For this review, take the finished solid that the model builds, in its own axes (mm). Face numbers are marked on the shaded views. Round coordinates to 2 decimals unless told otherwise and drop trailing zeros. Write each loop counter-clockwise with the first axis right and the second up, starting at its lowest first coordinate (ties: lowest second). Pieces come first, ordered by that corner, then holes. Notation, with made-up numbers: M 48,76 L 66,76 A8 cw 66,89 Z; hole C -5.75,56.5 d4. An arc over 180 degrees is marked long. Use one line per item in the form item = value. Start each with the question number.
Item 1: Add section C-C (z = 11). State the section outline as (x, y) points, and give its area (3 significant figures).
Item 2: For line 1 (Z direction, x = 0, y = 3.1); line 2 (Z direction, x = 10.75, y = -4); line 3 (X direction, y = 0.5, z = 0.5), list the stretches that pass through material, from the lowest coordinate up. Write a range as [from, to].
Item 3: Add section B-B (y = -15.5). State the section outline as (x, z) points, and give its area (3 significant figures).
Item 4: Add section A-A (x = 0). State the section outline as (y, z) points (3 decimals).
Item 5: Draft analysis for pull direction Z (two halves, no side actions). For the marked faces 1 and 2, state which applies: released by +Z, released by -Z, zero draft, split by the parting line, or undercut.
Item 6: For P1, Ø3, axis at x = -2, y = -6, coming from the +Z side; P2, Ø1.5, axis at x = 8.5, y = 6.5, coming from the +Z side; P3, Ø8, axis at x = -0.5, z = 17, coming from the -Y side, all flat-tipped, find the tip position at first contact; note any pin that passes through.
from build123d import *

# Parameters (mm, degrees)
F2_DEPTH = 3.175
F0_R     = 6.35
F3_DEPTH = 3.175
F4_DEPTH = 19.05
F0_W     = 6.35
F0_H     = 25.4
F6_DEPTH = 3.048


with BuildPart() as f1:
    # F0 (on Front) → F1 (revolve)
    with BuildSketch(Plane.XZ):
        Polygon((12.7, 93.701775), (0, 93.701775), (0, -7.898225), (6.35, -7.898225), (12.7, -7.898225), align=None)
    revolve(axis=Axis((0, 0, 42.901775), (0, 0, -1)))

    # F0 (on Front) → F2 (join, symmetric)
    with BuildSketch(Plane.XZ):
        with BuildLine():
            Line((-9.525, 144.402459), (-12.7, 93.701775))
            Line((-12.7, 93.701775), (0, 93.701775))
            Line((0, 93.701775), (12.7, 93.701775))
            Line((12.7, 93.701775), (9.525, 144.402459))
            ThreePointArc((9.525, 144.402459), (0, 134.877459), (-9.525, 144.402459))
        make_face()
    extrude(amount=F2_DEPTH, both=True)

    # F0 (on Front) → F3 (join, symmetric)
    with BuildSketch(Plane.XZ):
        with BuildLine():
            ThreePointArc((9.525, 144.402459), (0, 153.927459), (-9.525, 144.402459))
            ThreePointArc((-9.525, 144.402459), (0, 134.877459), (9.525, 144.402459))
        make_face()
        with Locations((0, 144.402459)):
            Circle(F0_R, mode=Mode.SUBTRACT)
    extrude(amount=F3_DEPTH, both=True)

    # F0 (on Front) → F4 (join)
    with BuildSketch(Plane.XZ):
        with Locations((0, 144.402459)):
            Circle(F0_R)
    extrude(amount=F4_DEPTH)

    # F0 (on Front) → F5 (revolve)
    with BuildSketch(Plane.XZ):
        with Locations((3.175, -20.598225)):
            Rectangle(F0_W, F0_H)
    revolve(axis=Axis((0, 0, -20.598225), (0, 0, -1)))

    # F0 (on Front) → F6 (join)
    with BuildSketch(Plane.XZ):
        with Locations((0, 144.402459)):
            Circle(F0_R)
    extrude(amount=-F6_DEPTH)


solid = f1.part
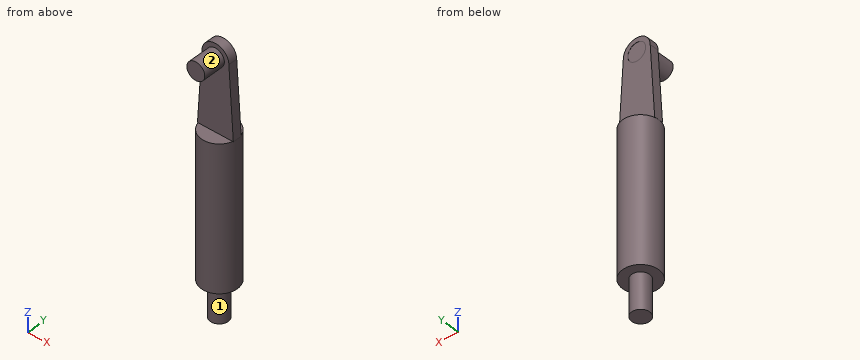
Calculated:
q1.outline = C 0,0 d25.4
q1.area = 507 mm^2
q2.line_1 = [-33.3, 138.05], [150.75, 153.93]
q2.line_2 = [-7.9, 93.7]
q2.line_3 = [-12.69, 12.69]
q3.outline = C 0,144.4 d12.7
q3.area = 127 mm^2
q4.outline = M -19.05,138.052 L -3.175,138.052 L -3.175,93.702 L -12.7,93.702 L -12.7,-7.898 L -6.35,-7.898 L -6.35,-33.298 L 6.35,-33.298 L 6.35,-7.898 L 12.7,-7.898 L 12.7,93.702 L 3.175,93.702 L 3.175,138.052 L 3.048,138.052 L 3.048,150.752 L 3.175,150.752 L 3.175,153.927 L -3.175,153.927 L -3.175,150.752 L -19.05,150.752 Z
q5.face_1 = zero draft
q5.face_2 = undercut
q6.P1 = 150.73
q6.P2 = 93.7
q6.P3 = -12.7
